```python
from build123d import *

# Parameters (mm, degrees)
SKETCH1_R           = 6.75
BOSS_EXTRUDE1_DEPTH = 88.9
CHAMFER1_SIZE       = 0.635
CUT_EXTRUDE1_DEPTH  = 12.7
CIRPATTERN2_COUNT   = 35


with BuildPart() as part:
    # Sketch1 → Boss-Extrude1 (new body)
    with BuildSketch(Plane(origin=(0, 0, 0), x_dir=(0, 0, -1), z_dir=(1, 0, 0))):
        Circle(SKETCH1_R)
    extrude(amount=BOSS_EXTRUDE1_DEPTH)

    # Chamfer1
    chamfer1_edges = [part.edges().sort_by_distance(p)[0] for p in [
        (88.9, 0, 6.75),
    ]]
    chamfer(chamfer1_edges, length=CHAMFER1_SIZE)

    # Sketch2 → Cut-Extrude1 (cut)
    with BuildSketch(Plane(origin=(88.9, 0, 0), x_dir=(0, 0, -1), z_dir=(1, 0, 0))):
        Polygon((-1.067952277, 7.359736044), (0, 6.291783767), (1.067952277, 7.359736044), align=None)
    cut_extrude1 = extrude(amount=-CUT_EXTRUDE1_DEPTH, mode=Mode.SUBTRACT)

    # CirPattern2: Cut-Extrude1 ×35 about axis
    cirpattern2_axis = Axis((0, 0, 0), (1, 0, 0))
    for i in range(1, CIRPATTERN2_COUNT):
        add(cut_extrude1.rotate(cirpattern2_axis, i * 360 / CIRPATTERN2_COUNT), mode=Mode.SUBTRACT)


solid = part.part
```
Read the model definition and answer for the solid it produces. Units are mm, in the model's axes. Round coordinates to 2 decimals unless told otherwise and drop trailing zeros. Loops run counter-clockwise (first coordinate to the right, second up) from the corner with the lowest first, then second, coordinate; pieces in that order, holes last. Notation, with made-up numbers: (6, 9.25) -> (28, 9.25) arc R28 cw to (28, 33.25) -> close; hole circle Ø2 at (-38, 21). An arc over 180 degrees is marked (long way). One line per item, written item: value.
1) Consider L1, parallel to Y at x = 64.5, z = 1.25; L2, parallel to Z at x = 8.5, y = -5; L3, parallel to Z at x = 23, y = -3.5. Determine where each line is inside the solid, lowest interval first. Write a range as [from, to].
Answer list:
L1: y = [-6.63, 6.63]
L2: z = [-4.53, 4.53]
L3: z = [-5.77, 5.77]
2) Flat-ended cylindrical pins translate along their axes: P1, Ø8, axis at x = 29, y = 1.5, coming from the +Z side; P2, Ø5, axis at x = 26.5, z = -5.5, coming from the -Y side; P3, Ø0.5, axis at y = 6.5, z = 0, coming from the +X side (3 decimals); P4, Ø1.5, axis at x = 62.5, z = -5, coming from the -Y side. Find the tip coordinate at first contact, or state that the pin passes through.
Answer list:
P1: stops at z = 6.75
P2: stops at y = -6.05
P3: stops at x = 88.765
P4: stops at y = -5.24
3) A cutting plane is placed at A-A (x = 6.5). Determine the outline of the cut face in (y, z).
Answer list:
outline: circle Ø13.5 at (0, 0)
